Read the model definition and answer for the solid it produces. Units are mm, in the model's axes. A direction names the side the tool comes from. Give positions to 0.01 mm unless a question says otherwise; leave off trailing zeros. Write each loop counter-clockwise with the first axis right and the second up, starting at its lowest first coordinate (ties: lowest second). Pieces come first, ordered by that corner, then holes. Notation, with made-up numbers: (-14, 2.25) - (-4, 2.25) arc R21 ccw to (-4, 11.25) - close; hole circle Ø5 at (70, 23.25). An arc over 180 degrees is marked (long way). Answer as a JSON object with one key per item and string values. Group by question number.
Autodesk Fusion 360 part; units mm, degrees
sketch "Sketch1" plane through (0, 0, 0) normal (1, 0, 0) x (0, 1, 0)
  line L0 (0, 0) -> (101.6, 0)
  line L1 (101.6, 0) -> (101.6, 38.1)
  line L2 (101.6, 38.1) -> (0, 38.1)
  line L3 (0, 38.1) -> (0, 0)
  line L4 (0, 0) -> (0, -3.175)
  line L5 (0, -3.175) -> (12.7, -3.175)
  line L6 (12.7, -3.175) -> (12.7, 0)
  line L7 (12.7, 0) -> (25.4, 0)
  line L8 (25.4, 0) -> (25.4, -3.175)
  line L9 (25.4, -3.175) -> (38.1, -3.175)
  line L10 (38.1, -3.175) -> (38.1, 0)
  line L11 (101.6, 0) -> (101.6, -3.175)
  line L12 (101.6, -3.175) -> (88.9, -3.175)
  line L13 (88.9, -3.175) -> (88.9, 0)
  line L14 (88.9, 0) -> (76.2, 0)
  line L15 (76.2, 0) -> (76.2, -3.175)
  line L16 (76.2, -3.175) -> (63.5, -3.175)
  line L17 (63.5, -3.175) -> (63.5, 0)
  line L18 (101.6, 0) -> (104.775, 0)
  line L19 (104.775, 0) -> (104.775, 12.7)
  line L20 (104.775, 12.7) -> (101.6, 12.7)
  line L21 (101.6, 38.1) -> (104.775, 38.1)
  line L22 (104.775, 38.1) -> (104.775, 25.4)
  line L23 (104.775, 25.4) -> (101.6, 25.4)
  line L24 (0, 38.1) -> (-3.175, 38.1)
  line L25 (-3.175, 38.1) -> (-3.175, 25.4)
  line L26 (-3.175, 25.4) -> (0, 25.4)
  line L27 (0, 0) -> (-3.175, 0)
  line L28 (-3.175, 0) -> (-3.175, 12.7)
  line L29 (-3.175, 12.7) -> (0, 12.7)
  dimension "d1" = 101.6
  dimension "d2" = 38.1
  dimension "d3" = 3.175
  dimension "d4" = 12.7
  dimension "d5" = 12.7
  dimension "d6" = 3.175
  dimension "d7" = 12.7
  dimension "d8" = 3.175
  dimension "d9" = 12.7
  dimension "d10" = 12.7
  dimension "d11" = 3.175
  dimension "d12" = 12.7
  dimension "d13" = 3.175
  dimension "d14" = 12.7
  dimension "d15" = 3.175
  dimension "d16" = 12.7
  dimension "d17" = 3.175
  dimension "d18" = 12.7
  dimension "d19" = 3.175
  dimension "d20" = 12.7
extrude "Extrude1" add sketch "Sketch1" along normal blind 3.175
sketch "Sketch2" plane through (3.175, 0, 0) normal (1, 0, 0) x (0, 1, 0)
  line L0 (0, 0) -> (0, -3.175)
  line L1 (0, -3.175) -> (12.7, -3.175)
  line L2 (12.7, -3.175) -> (12.7, 0)
  line L3 (12.7, 0) -> (25.4, 0)
  line L4 (25.4, 0) -> (25.4, -3.175)
  line L5 (25.4, -3.175) -> (38.1, -3.175)
  line L6 (38.1, -3.175) -> (38.1, 0)
  line L7 (38.1, 0) -> (63.5, 0)
  line L8 (63.5, 0) -> (63.5, -3.175)
  line L9 (63.5, -3.175) -> (76.2, -3.175)
  line L10 (76.2, -3.175) -> (76.2, 0)
  line L11 (76.2, 0) -> (88.9, 0)
  line L12 (88.9, 0) -> (88.9, -3.175)
  line L13 (88.9, -3.175) -> (101.6, -3.175)
  line L14 (101.6, -3.175) -> (101.6, 0)
  line L15 (101.6, 0) -> (104.775, 0)
  line L16 (104.775, 0) -> (104.775, 12.7)
  line L17 (104.775, 12.7) -> (101.6, 12.7)
  line L18 (101.6, 12.7) -> (101.6, 25.4)
  line L19 (101.6, 25.4) -> (104.775, 25.4)
  line L20 (104.775, 25.4) -> (104.775, 38.1)
  line L21 (104.775, 38.1) -> (-3.175, 38.1)
  line L22 (-3.175, 38.1) -> (-3.175, 25.4)
  line L23 (-3.175, 25.4) -> (0, 25.4)
  line L24 (0, 25.4) -> (0, 12.7)
  line L25 (0, 12.7) -> (-3.175, 12.7)
  line L26 (-3.175, 12.7) -> (-3.175, 0)
  line L27 (-3.175, 0) -> (0, 0)
  line L28 (50.8, 0) -> (63.5, 0)
  line L29 (63.5, 0) -> (63.5, -3.175)
  line L30 (63.5, -3.175) -> (76.2, -3.175)
  line L31 (76.2, -3.175) -> (76.2, 0)
  line L32 (76.2, 0) -> (88.9, 0)
  line L33 (88.9, -3.175) -> (88.9, 0)
  line L34 (88.9, -3.175) -> (101.6, -3.175)
  line L35 (101.6, -3.175) -> (101.6, 0)
  line L36 (104.775, 0) -> (104.775, 12.7)
  line L37 (104.775, 12.7) -> (101.6, 12.7)
  line L38 (101.6, 12.7) -> (101.6, 25.4)
  line L39 (104.775, 25.4) -> (104.775, 38.1)
  line L40 (104.775, 38.1) -> (50.8, 38.1)
  line L41 (63.5, 0) -> (57.15, 0)
  line L42 (50.8, 38.1) -> (53.975, 38.1)
  line L43 (53.975, 38.1) -> (57.15, 38.1)
  line L44 (57.15, 38.1) -> (57.15, 0)
  line L45 (57.15, 38.1) -> (57.15, 0)
  line L46 (25.4, -3.175) -> (12.7, -3.175)
  line L47 (9.525, 25.4) -> (9.525, 38.1)
  line L48 (9.525, 12.7) -> (12.7, 12.7)
  line L49 (12.7, 12.7) -> (12.7, 25.4)
  line L50 (9.525, 0) -> (9.525, 12.7)
  line L51 (12.7, -3.175) -> (12.7, 0)
  line L52 (12.7, 0) -> (9.525, 0)
  line L53 (12.7, 25.4) -> (9.525, 25.4)
  line L54 (9.525, 12.7) -> (12.7, 12.7)
  line L55 (50.8, -3.175) -> (38.1, -3.175)
  line L56 (9.525, 0) -> (9.525, 12.7)
  line L57 (9.525, 25.4) -> (9.525, 38.1)
  line L58 (38.1, 0) -> (25.4, 0)
  line L59 (38.1, -3.175) -> (38.1, 0)
  line L60 (50.8, 0) -> (50.8, -3.175)
  line L61 (12.7, -3.175) -> (12.7, 0)
  line L62 (25.4, 0) -> (25.4, -3.175)
  line L63 (50.8, 0) -> (50.8, -3.175)
  line L64 (50.8, -3.175) -> (38.1, -3.175)
  line L65 (38.1, -3.175) -> (38.1, 0)
  line L66 (25.4, -3.175) -> (25.4, 0)
  line L67 (25.4, -3.175) -> (12.7, -3.175)
  line L68 (12.7, 12.7) -> (12.7, 25.4)
  line L69 (38.1, 0) -> (25.4, 0)
  line L70 (50.8, -3.175) -> (63.5, -3.175)
  point P0 (50.8, 0)
  dimension "d23" = 3.175
  dimension "d24" = 3.175
extrude "Extrude5" add sketch "Sketch2" against normal blind 3.175 contours L6 L7 L55 L59 L60 L63 L64 L65 | L7 L8 L28 L29 L41 L60 L63 L70
extrude "Extrude3" cut sketch "Sketch2" against normal blind 30.48 contours L0 L1 L2 L21 L22 L23 L24 L25 L26 L27 L47 L48 L49 L50 L51 L52 L53 L54 L56 L57 L61 L68
extrude "Extrude2" cut sketch "Sketch2" against normal blind 15.24 contours L0 L1 L2 L21 L22 L23 L24 L25 L26 L27 L47 L48 L49 L50 L51 L52 L53 L54 L56 L57 L61 L68 | L3 L7 L21 L28 L40 L42 L43 L44 L45 L47 L48 L49 L50 L52 L53 L54 L56 L57 L58 L68 L69 | L4 L5 L6 L58 L59 L62 L65 L66 L69
extrude "Extrude4" add sketch "Sketch2" against normal blind 3.175 contours L2 L3 L4 L46 L51 L61 L62 L66 L67 | L3 L7 L21 L28 L40 L42 L43 L44 L45 L47 L48 L49 L50 L52 L53 L54 L56 L57 L58 L68 L69 | L6 L7 L55 L59 L60 L63 L64 L65
sketch "Sketch3" plane through (3.175, 0, 0) normal (1, 0, 0) x (0, 1, 0)
  line L0 (38.1, -3.175) -> (76.2, -3.175)
  line L1 (76.2, -3.175) -> (76.2, 0)
  line L2 (76.2, 0) -> (88.9, 0)
  line L3 (88.9, 0) -> (88.9, -3.175)
  line L4 (88.9, -3.175) -> (101.6, -3.175)
  line L5 (101.6, -3.175) -> (101.6, 0)
  line L6 (101.6, 0) -> (104.775, 0)
  line L7 (104.775, 0) -> (104.775, 12.7)
  line L8 (104.775, 12.7) -> (101.6, 12.7)
  line L9 (101.6, 12.7) -> (101.6, 25.4)
  line L10 (101.6, 25.4) -> (104.775, 25.4)
  line L11 (104.775, 25.4) -> (104.775, 38.1)
  line L12 (104.775, 38.1) -> (9.525, 38.1)
  line L13 (9.525, 38.1) -> (9.525, 25.4)
  line L14 (9.525, 25.4) -> (12.7, 25.4)
  line L15 (12.7, 25.4) -> (12.7, 12.7)
  line L16 (12.7, 12.7) -> (9.525, 12.7)
  line L17 (9.525, 12.7) -> (9.525, 0)
  line L18 (9.525, 0) -> (12.7, 0)
  line L19 (12.7, 0) -> (12.7, -3.175)
  line L20 (12.7, -3.175) -> (25.4, -3.175)
  line L21 (25.4, -3.175) -> (25.4, 0)
  line L22 (25.4, 0) -> (38.1, 0)
  line L23 (38.1, 0) -> (38.1, -3.175)
  line L24 (12.7, 0) -> (12.7, -3.175)
  line L25 (12.7, -3.175) -> (25.4, -3.175)
  line L26 (25.4, -3.175) -> (25.4, 0)
  line L27 (38.1, 0) -> (25.4, 0)
  line L28 (38.1, 0) -> (38.1, -3.175)
  line L29 (38.1, -3.175) -> (76.2, -3.175)
  line L30 (76.2, 0) -> (76.2, -3.175)
  line L31 (76.2, 0) -> (88.9, 0)
  line L32 (88.9, -3.175) -> (88.9, 0)
  line L33 (88.9, -3.175) -> (101.6, -3.175)
  line L34 (101.6, -3.175) -> (101.6, 0)
  line L35 (101.6, 0) -> (104.775, 0)
  line L36 (104.775, 0) -> (104.775, 12.7)
  line L37 (104.775, 12.7) -> (101.6, 12.7)
  line L38 (101.6, 12.7) -> (101.6, 25.4)
  line L39 (101.6, 25.4) -> (104.775, 25.4)
  line L40 (104.775, 25.4) -> (104.775, 38.1)
  line L41 (104.775, 38.1) -> (9.525, 38.1)
  line L42 (9.525, 38.1) -> (9.525, 25.4)
  line L43 (9.525, 25.4) -> (12.7, 25.4)
  line L44 (12.7, 25.4) -> (12.7, 12.7)
  line L45 (12.7, 12.7) -> (9.525, 12.7)
  line L46 (9.525, 12.7) -> (9.525, 0)
  line L47 (9.525, 0) -> (12.7, 0)
sketch "Sketch4" plane through (3.175, 0, 0) normal (1, 0, 0) x (0, 1, 0)
  line L0 (38.1, -3.175) -> (76.2, -3.175)
  line L1 (76.2, -3.175) -> (76.2, 0)
  line L2 (76.2, 0) -> (88.9, 0)
  line L3 (88.9, 0) -> (88.9, -3.175)
  line L4 (88.9, -3.175) -> (101.6, -3.175)
  line L5 (101.6, -3.175) -> (101.6, 0)
  line L6 (101.6, 0) -> (104.775, 0)
  line L7 (104.775, 0) -> (104.775, 12.7)
  line L8 (104.775, 12.7) -> (101.6, 12.7)
  line L9 (101.6, 12.7) -> (101.6, 25.4)
  line L10 (101.6, 25.4) -> (104.775, 25.4)
  line L11 (104.775, 25.4) -> (104.775, 38.1)
  line L12 (104.775, 38.1) -> (9.525, 38.1)
  line L13 (9.525, 38.1) -> (9.525, 25.4)
  line L14 (9.525, 25.4) -> (12.7, 25.4)
  line L15 (12.7, 25.4) -> (12.7, 12.7)
  line L16 (12.7, 12.7) -> (9.525, 12.7)
  line L17 (9.525, 12.7) -> (9.525, 0)
  line L18 (9.525, 0) -> (12.7, 0)
  line L19 (12.7, 0) -> (12.7, -3.175)
  line L20 (12.7, -3.175) -> (25.4, -3.175)
  line L21 (25.4, -3.175) -> (25.4, 0)
  line L22 (25.4, 0) -> (38.1, 0)
  line L23 (38.1, 0) -> (38.1, -3.175)
  line L24 (101.6, 12.7) -> (104.775, 12.7)
  line L25 (104.775, 25.4) -> (104.775, 12.7)
  line L26 (104.775, 25.4) -> (101.6, 25.4)
  line L27 (101.6, 25.4) -> (101.6, 12.7)
  line L28 (101.6, 25.4) -> (101.6, 38.1)
  line L29 (101.6, 38.1) -> (104.775, 38.1)
  line L30 (104.775, 38.1) -> (104.775, 0)
  line L31 (104.775, 0) -> (101.6, 0)
  line L32 (101.6, 0) -> (101.6, 25.4)
extrude "Extrude7" cut sketch "Sketch4" against normal blind 5.08 contours L6 L7 L8 L24 L30 L31 L32 | L10 L11 L12 L26 L28 L29 L30
extrude "Extrude6" cut sketch "Sketch4" against normal blind 20.32 contours L6 L7 L8 L24 L30 L31 L32 | L10 L11 L12 L26 L28 L29 L30
extrude "Extrude8" add sketch "Sketch4" against normal blind 3.175 contours L8 L9 L10 L24 L25 L26 L27 L30 L32
1) Find section C-C, the plane z = 15. Write down the section's boundary in (x, y) (3 decimals).
2) Find section B-B, the plane y = 80. Write down the section's boundary in (x, z) (3 decimals), and give its area (3 significant figures).
3) Find section A-A, the plane x = 1.8. Write down the section's boundary in (y, z) (3 decimals).
4) For a pull along Y with two mould halves and no side action, classify faces 4 (the flat face through (2, 57, -3.175)), 5 (the flat face through (2, 12.7, -2)), 6 (the flat face through (2, 32, 0)) as released by +Y, released by -Y, zero draft, split by the parting line, or undercut.
5) Flat-ended cylindrical pins translate along their axes: pin 1 Ø1 at (x, z) = (1.5, 34) entering from +Y; pin 2 Ø1 at (x, z) = (1, 21.5) entering from -Y; pin 3 Ø1.6 at (x, y) = (2, 103.5) entering from -Z. Find the tip coordinate at first contact, or state that the pin passes through.
6) Which of the six approach directions +Z, -Z, +X, -X, +Y, -Y give full straight-line access (tool end or side, diameter ignored) to faces 1 (the flat face through (2, 101.6, 32)), 2 (the flat face through (2, 12.7, 19)), 3 (the flat face through (2, 76.2, -2))?
7) Find the intervals of material crossed by line 1 (Y direction, x = 1.55, z = -1); line 2 (Z direction, x = 2.25, y = 79.5); line 3 (Y direction, x = 2.8, z = 18) (3 decimals), in increasing order. Write a range as [from, to].
Values follow:
{
 "1": {"outline": "(0, 12.7) - (3.175, 12.7) - (3.175, 104.775) - (0, 104.775) - close"},
 "2": {"outline": "(0, 0) - (3.175, 0) - (3.175, 38.1) - (0, 38.1) - close", "area": "121 mm2"},
 "3": {"outline": "(9.525, 0) - (12.7, 0) - (12.7, -3.175) - (25.4, -3.175) - (25.4, 0) - (38.1, 0) - (38.1, -3.175) - (76.2, -3.175) - (76.2, 0) - (88.9, 0) - (88.9, -3.175) - (101.6, -3.175) - (101.6, 12.7) - (104.775, 12.7) - (104.775, 25.4) - (101.6, 25.4) - (101.6, 38.1) - (9.525, 38.1) - (9.525, 25.4) - (12.7, 25.4) - (12.7, 12.7) - (9.525, 12.7) - close"},
 "4": {"face 4": "zero draft", "face 5": "released by -Y", "face 6": "undercut"},
 "5": {"pin 1": "stops at y = 101.6", "pin 2": "stops at y = 12.7", "pin 3": "stops at z = 12.7"},
 "6": {"face 1": "+Z, +X, -X, +Y", "face 2": "+X, -X, -Y", "face 3": "-Z, +X, -X"},
 "7": {"line 1": "y = [12.7, 25.4], [38.1, 76.2], [88.9, 101.6]", "line 2": "z = [0, 38.1]", "line 3": "y = [12.7, 104.775]"}
}
